Here's the drawing with two shaded views (mm, measured from the low corner). I have some questions. A direction names the side the tool comes from. Coordinates: 2 decimals unless noted, no trailing zeros. Write each loop counter-clockwise with the first axis right and the second up, starting at its lowest first coordinate (ties: lowest second). Pieces come first, ordered by that corner, then holes.
Item 1: We'd pull the mould along X, two halves only. Please class the marked faces 1, 2 and 3: +X half, -X half, draft (parallel to the pull), parting line (faces both ways), or undercut.
Item 2: If we section it at A-A (x = 1836): Please give me the cut outline in (y, z).
Item 3: If we section it at B-B (y = 375.5): Please give me the cut outline in (x, z).
Item 4: For the marked faces 4 and 5, which set-ups out of +Z, -Z, +X, -X, +Y, -Y let a thin tool reach every point of the face, with its end or its side?
Item 5: If I drill on line 1 (Y direction, x = 1784, z = 90); line 2 (X direction, y = 67, z = 440.5), over which ranges is the centre line in solid material (lowest first)?
Item 6: If we section it at C-C (z = 265.5): Count the separate pieces of the cut face and the enclosed holes in it, then the cut area to 3 significant figures.
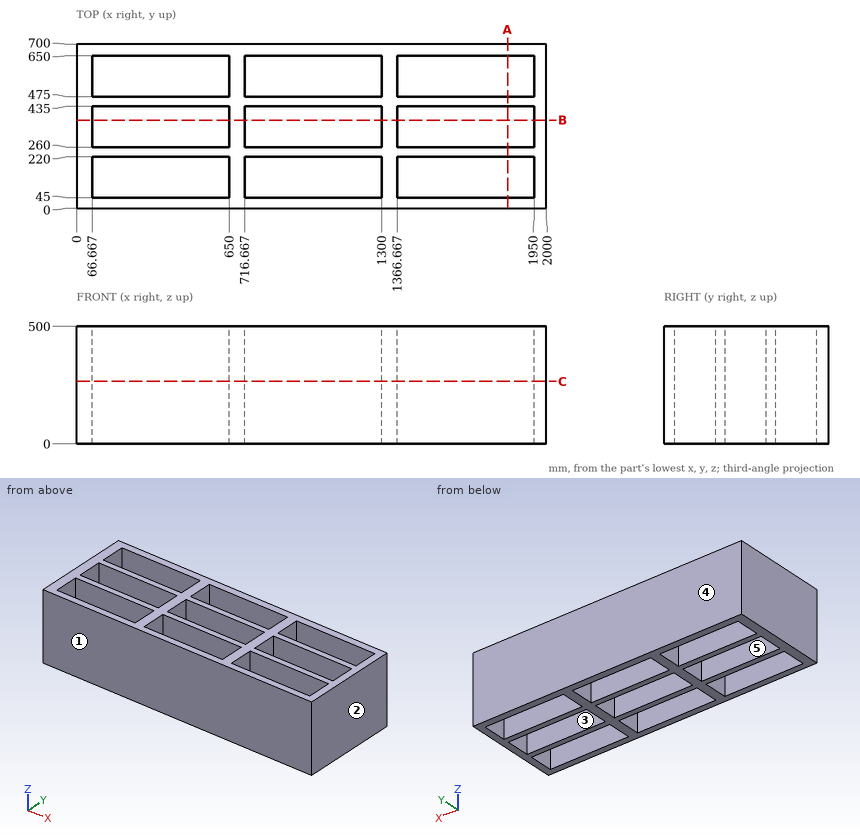
Answer list:
1. face 1: draft
1. face 2: +X half
1. face 3: undercut
2. outline: (0, 0) - (45, 0) - (45, 500) - (0, 500) - close; (220, 0) - (260, 0) - (260, 500) - (220, 500) - close; (435, 0) - (475, 0) - (475, 500) - (435, 500) - close; (650, 0) - (700, 0) - (700, 500) - (650, 500) - close
3. outline: (0, 0) - (66.67, 0) - (66.67, 500) - (0, 500) - close; (650, 0) - (716.67, 0) - (716.67, 500) - (650, 500) - close; (1300, 0) - (1366.67, 0) - (1366.67, 500) - (1300, 500) - close; (1950, 0) - (2000, 0) - (2000, 500) - (1950, 500) - close
4. face 4: +Z, -Z, +X, -X, +Y
4. face 5: +Z, -Z
5. line 1: y = 0 to 45, 220 to 260, 435 to 475, 650 to 700
5. line 2: x = 0 to 66.67, 650 to 716.67, 1300 to 1366.67, 1950 to 2000
6. separate pieces: 1
6. enclosed holes: 9
6. area: 481,000 mm2
